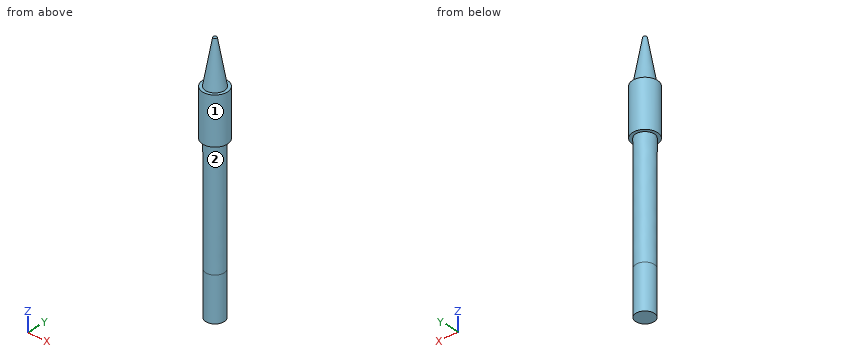
```python
from build123d import *

# Parameters (mm, degrees)
SKETCH1_R           = 6.225
BOSS_EXTRUDE1_DEPTH = 80
BOSS_EXTRUDE1_DRAFT = -0.08
SKETCH1_2_R         = 6.225
BOSS_EXTRUDE2_DEPTH = 30
SKETCH2_R           = 8.5
BOSS_EXTRUDE3_DEPTH = 32
SKETCH3_R           = 6.5
BOSS_EXTRUDE4_DEPTH = 30
BOSS_EXTRUDE4_TAPER = 10


with BuildPart() as part:
    # Sketch1 → Boss-Extrude1 (with draft: the straight prism first)
    with BuildSketch(Plane.XY):
        Circle(SKETCH1_R)
    extrude(amount=BOSS_EXTRUDE1_DEPTH)
    # Boss-Extrude1: the draft: its side faces are tilted about the plane it starts from
    boss_extrude1_sides = [part.faces().sort_by_distance(p)[0] for p in [
        (-6.225, 0, 40),
    ]]
    draft(boss_extrude1_sides, Plane.XY, BOSS_EXTRUDE1_DRAFT)

    # Sketch1<2> → Boss-Extrude2 (add)
    with BuildSketch(Plane.XY):
        Circle(SKETCH1_2_R)
    extrude(amount=-BOSS_EXTRUDE2_DEPTH)

    # Sketch2 → Boss-Extrude3 (add)
    with BuildSketch(Plane.XY.offset(80)):
        Circle(SKETCH2_R)
    extrude(amount=BOSS_EXTRUDE3_DEPTH)

    # Sketch3 → Boss-Extrude4 (add)
    with BuildSketch(Plane.XY.offset(112)):
        Circle(SKETCH3_R)
    extrude(amount=BOSS_EXTRUDE4_DEPTH, taper=BOSS_EXTRUDE4_TAPER)


solid = part.part
```
Design review of the part built by this model. Coordinates are the model's own, in mm. Face numbers are marked on the shaded views. A direction names the side the tool comes from. Give positions to 0.01 mm unless a question says otherwise; leave off trailing zeros. Order: outer loops, then holes, each group sorted by start corner. A loop starts at its lowest first (then second) coordinate and runs counter-clockwise, first axis right, second up. Notation, with made-up numbers: M -20.75,15 L -4.75,15 A10 ccw -4.75,26 Z; hole C 70.5,70.5 d4. An arc over 180 degrees is marked long. One line per question, with ' | ' between items. Start each with the question number.
Q1. We need section A-A (z = 69). Write out the cut boundary in (x, y).
Q2. For pin 1 Ø2 at (y, z) = (-2.5, 113.5) entering from -X; pin 2 Ø1.5 at (x, z) = (-3, 105) entering from -Y; pin 3 Ø1 at (x, z) = (-4.5, -11) entering from -Y, all flat-tipped, find the tip position at first contact; note any pin that passes through.
Q3. Machinability: for the marked faces 1 and 2, which of the approach directions +Z, -Z, +X, -X, +Y, -Y give a long, thin tool a straight path to every point of the face, cutting with its end or side? Answer none if there is none.
Q4. For L1, parallel to Y at x = 1, z = 71; L2, parallel to Z at x = 4.75, y = 4.75; L3, parallel to Y at x = 0.25, z = 106, list the stretches that pass through material, from the lowest coordinate up. Write a range as [from, to].
Q5. We need section B-B (z = 19.5). Write out the cut boundary in (x, y).
Returned:
1) outline: C 0,0 d12.64
2) pin 1: x = -6.11 | pin 2: y = -8.2 | pin 3: y = -4.77
3) face 1: +Z, -Z | face 2: -Z
4) L1: [-6.24, 6.24] | L2: [80, 112] | L3: [-8.5, 8.5]
5) outline: C 0,0 d12.5
